Input: part model. Units: mm. Frame: model coordinates. A direction names the side the tool comes from. Coordinates: 2 decimals unless noted, no trailing zeros. Order: outer loops, then holes, each group sorted by start corner. A loop starts at its lowest first (then second) coordinate and runs counter-clockwise, first axis right, second up. Notation, with made-up numbers: (-17.5, 40.25) - (33.5, 40.25) arc R14 cw to (33.5, 55.25) - close; hole circle Ø11 at (61.5, 38.5). An arc over 180 degrees is marked (long way). Answer as CSV lines item,"result". Start each with the question number.
Item 1: Section C-C (z = 1499). Output: boundary loops of the cut face in (x, y), and give its area (3 significant figures).
Item 2: Section A-A (x = 896.5). Output: boundary loops of the cut face in (y, z) (3 decimals), and give its area (3 significant figures).
Item 3: Draft query along Y for faces 1 (the flat face through (1000, 850, 840)), 2 (the flat face through (542, 507, 0)), 3 (the flat face through (546, 900, 49)). Return one class per face: +Y half, -Y half, draft (parallel to the pull), parting line (faces both ways), or undercut.
Item 4: Section B-B (x = 349). Output: boundary loops of the cut face in (y, z) (3 decimals), and give its area (3 significant figures).
Item 5: First-contact query: pin 1 (2 mm diameter, centred on x = 795, z = 531.5, fed in from +Y). Flat tip, straight axial feed; report the tip coordinate or a pass-through.
Item 6: Section D-D (y = 937.5). Output: boundary loops of the cut face in (x, z), and give its area (3 significant figures).
Item 7: Access query for faces 4 (the flat face through (1049, 1200, 1279)), 5 (the flat face through (295, 1008, 51)), 6 (the flat face through (80, 1200, 593)). Directions: +Z, -Z, +X, -X, +Y, -Y. A direction counts if a zero-diameter tool reaches every point of the face in a straight line with its end or side. Return the directions, or none.
Item 8: Material intervals for line 1 along Z through (x, y) = (529, 517); line 2 along Y through (x, z) = (185.5, 950); line 3 along X through (y, z) = (644.5, 1309), sorted ascending.
Autodesk Inventor part; units mm, degrees
ref_plane "YZ Plane" through (0, 0, 0) normal (1, 0, 0) x (0, 1, 0)
ref_plane "XZ Plane" through (0, 0, 0) normal (0, 1, 0) x (-1, 0, 0)
ref_plane "XY Plane" through (0, 0, 0) normal (0, 0, 1) x (1, 0, 0)
sketch "Sketch10" plane through (0, 0, 0) normal (0, 1, 0) x (-1, 0, 0)
  point P0 (0, 0)
sketch "Sketch11" plane through (0, 0, 0) normal (0, 0, 1) x (1, 0, 0)
  point P0 (0, 0)
sketch "Sketch12" plane through (0, 0, 0) normal (0, 0, 1) x (1, 0, 0)
  line L0 (0, 0) -> (1100, 0)
  line L1 (1100, 0) -> (1100, 1200)
  line L2 (1100, 1200) -> (0, 1200)
  line L3 (0, 1200) -> (0, 0)
  dimension "d20" = 1100
  dimension "d21" = 1200
extrude "Extrusion6" add sketch "Sketch12" along normal blind 1700
sketch "Sketch13" plane through (1100, 0, 0) normal (1, 0, 0) x (0, 0, -1)
  line L0 (-100, 100) -> (-1600, 100)
  line L1 (-1600, 100) -> (-1600, 1200)
  line L2 (-1600, 1200) -> (-100, 1200)
  line L3 (-100, 1200) -> (-100, 100)
  point P0 (0, 0)
  dimension "d24" = 1500
extrude "Extrusion7" cut sketch "Sketch13" against normal blind 1000
sketch "Sketch16" plane through (100, 0, 0) normal (1, 0, 0) x (0, 0, -1)
  circle A0 centre (-1499, 200) radius 50
  circle A1 centre (-201, 200) radius 50
  point P0 (0, 0)
  dimension "d34" = 100
  dimension "d35" = 100
extrude "Extrusion10" cut sketch "Sketch16" along normal blind 1200 and the other way blind 200
sketch "Sketch18" plane through (1100, 100, 100) normal (0, 0, 1) x (1, 0, 0)
  line L0 (0, 0) -> (-1000, 0)
  line L1 (-1000, 1100) -> (0, 1100)
  line L2 (0, 0) -> (-100, 0)
  line L3 (-100, 0) -> (-100, 1100)
  line L4 (-100, 1100) -> (0, 1100)
  line L5 (0, 1100) -> (0, 0)
  point P0 (-1100, -100)
  dimension "d43" = 100
extrude "Extrusion12" add sketch "Sketch18" along normal blind 1500
sketch "Sketch19" plane through (0, 0, 1700) normal (0, 0, 1) x (1, 0, 0)
  line L0 (100, 500) -> (1000, 500)
  line L1 (1000, 500) -> (1000, 510)
  line L2 (1000, 510) -> (100, 510)
  line L3 (100, 510) -> (100, 500)
  point P0 (0, 0)
  dimension "d46" = 900
  dimension "d47" = 10
extrude "Extrusion13" add sketch "Sketch19" against normal blind 1700
sketch "Sketch20" plane through (0, 0, 0) normal (0, 0, -1) x (-1, 0, 0)
  line L0 (-805, 1200) -> (-295, 1200)
  line L1 (-295, 1200) -> (-295, 900)
  line L2 (-295, 900) -> (-805, 900)
  line L3 (-805, 900) -> (-805, 1200)
  point P0 (0, 0)
  dimension "d58" = 510
  dimension "d59" = 300
extrude "Extrusion14" cut sketch "Sketch20" against normal blind 1700
sketch "Sketch21" plane through (1100, 1200, 1700) normal (0, 1, 0) x (1, 0, 0)
  line L0 (0, 1700) -> (0, 0)
  line L1 (-1100, 1700) -> (-1100, 0)
  line L2 (0, 470.5254) -> (-1100, 470.5254)
  line L3 (-1100, 470.5254) -> (-1100, 370.5254)
  line L4 (-1100, 370.5254) -> (0, 370.5254)
  line L5 (0, 370.5254) -> (0, 470.5254)
  dimension "d60" = 100
extrude "Extrusion15" add sketch "Sketch21" along normal blind 40
sketch "Sketch22" plane through (1100, 1240, 1700) normal (0, 1, 0) x (1, 0, 0)
  line L0 (-1100, 470.5254) -> (-1100, 370.5254)
  line L1 (0, 370.5254) -> (0, 470.5254)
  line L2 (-1100, 450.525) -> (0, 450.525)
  line L3 (0, 450.525) -> (0, 390.525)
  line L4 (0, 390.525) -> (-1100, 390.525)
  line L5 (-1100, 390.525) -> (-1100, 450.525)
  point P0 (-1100, 1700)
  dimension "d63" = 60
extrude "Extrusion16" cut sketch "Sketch22" against normal blind 40
sketch "Sketch23" plane through (1100, 1240, 1700) normal (0, 1, 0) x (1, 0, 0)
  point P0 (-1100, 1700)
sketch "Sketch25" plane through (1100, 0, 0) normal (1, 0, 0) x (0, 0, -1)
  point P0 (0, 0)
sketch "Sketch27" plane through (0, 0, 0) normal (0, 0, -1) x (-1, 0, 0)
  line L0 (-865, 700) -> (-785, 700)
  line L1 (-785, 700) -> (-785, 600)
  line L2 (-785, 600) -> (-865, 600)
  line L3 (-865, 600) -> (-865, 700)
  line L4 (0, 0) -> (-1100, 0)
  line L5 (-1100, 0) -> (-1100, 1200)
  line L6 (-805, 900) -> (-805, 1200)
  line L7 (-315, 700) -> (-235, 700)
  line L8 (-235, 700) -> (-235, 600)
  line L9 (-235, 600) -> (-315, 600)
  line L10 (-315, 600) -> (-315, 700)
  line L11 (-295, 1200) -> (-295, 900)
  dimension "d77" = 100
  dimension "d78" = 80
  dimension "d79" = 600
  dimension "d81" = 20
  dimension "d82" = 100
  dimension "d83" = 80
  dimension "d84" = 600
  dimension "d85" = 20
extrude "Extrusion17" cut sketch "Sketch27" against normal blind 10
sketch "Sketch28" plane through (0, 1200, 1229.4746) normal (0, 1, 0) x (1, 0, 0)
  line L0 (100, 0) -> (100, 1129.4746)
  line L1 (295, 1129.4746) -> (100, 1129.4746)
  line L2 (100, 1129.4746) -> (100, 878.7986)
  line L3 (100, 878.7986) -> (295, 878.7986)
  line L4 (295, 878.7986) -> (295, 1129.4746)
  point P0 (0, 1229.4746)
  point P1 (100, 1029.4746)
  dimension "d90" = 250.676
extrude "Extrusion18" add sketch "Sketch28" against normal blind 10
sketch "Sketch29" plane through (805, 1200, 0) normal (0, 1, 0) x (1, 0, 0)
  line L0 (0, 0) -> (0, -100)
  line L1 (195, -100) -> (195, -1229.4746)
  line L2 (0, -100) -> (195, -100)
  line L3 (195, -100) -> (195, -350.676)
  line L4 (195, -350.676) -> (0, -350.676)
  line L5 (0, -350.676) -> (0, -100)
  point P0 (-805, 0)
  dimension "d93" = 250.676
extrude "Extrusion19" add sketch "Sketch29" against normal blind 10
sketch "Sketch30" plane through (0, 1200, 0) normal (0, 1, 0) x (1, 0, 0)
  point P0 (0, 0)
fillet "Fillet3" radius 200 2 edges at (952.5, 1200, 0) (147.5, 1200, 0)
sketch "Sketch31" plane through (0, 0, 1700) normal (-1, 0, 0) x (0, 0, 1)
  circle A0 centre (-1499, 200) radius 50
  circle A1 centre (-1499, 200) radius 50
  point P0 (-1700, 0)
extrude "Extrusion20" cut sketch "Sketch31" against normal blind 10000
sketch "Sketch32" plane through (0, 0, 1700) normal (-1, 0, 0) x (0, 0, 1)
  circle A0 centre (-201, 200) radius 50
  circle A1 centre (-201, 200) radius 50
  point P0 (-1700, 0)
extrude "Extrusion21" cut sketch "Sketch32" against normal blind 10000
properties part number "Design" material "Copper"
Determined:
1,outline,"(0, 0) - (1100, 0) - (1100, 150) - (1000, 150) - (1000, 100) - (100, 100) - (100, 150) - (0, 150) - close; (0, 250) - (100, 250) - (100, 500) - (1000, 500) - (1000, 250) - (1100, 250) - (1100, 1200) - (1000, 1200) - (1000, 510) - (100, 510) - (100, 1200) - (0, 1200) - close"
1,area,"319,000 mm^2"
2,outline,"(0, 0) - (1000, 0) arc R200 ccw to (1173.205, 100) - (510, 100) - (510, 1600) - (1200, 1600) - (1200, 1700) - (0, 1700) - close; (1190, 137.55) arc R200 ccw to (1200, 200) - (1200, 350.676) - (1190, 350.676) - close; (1200, 1229.475) - (1240, 1229.475) - (1240, 1249.475) - (1200, 1249.475) - close; (1200, 1309.475) - (1240, 1309.475) - (1240, 1329.475) - (1200, 1329.475) - close; hole (100, 100) - (500, 100) - (500, 1600) - (100, 1600) - close"
2,area,"401,000 mm^2"
3,face 1,"undercut"
3,face 2,"draft"
3,face 3,"+Y half"
4,outline,"(0, 0) - (900, 0) - (900, 100) - (510, 100) - (510, 1600) - (900, 1600) - (900, 1700) - (0, 1700) - close; (1200, 1229.475) - (1240, 1229.475) - (1240, 1249.475) - (1200, 1249.475) - close; (1200, 1309.475) - (1240, 1309.475) - (1240, 1329.475) - (1200, 1329.475) - close; hole (100, 100) - (500, 100) - (500, 1600) - (100, 1600) - close"
4,area,"347,000 mm^2"
5,pin 1,"stops at y = 510"
6,outline,"(0, 0) - (295, 0) - (295, 100) - (100, 100) - (100, 1600) - (295, 1600) - (295, 1700) - (0, 1700) - close; (805, 0) - (1100, 0) - (1100, 1700) - (805, 1700) - (805, 1600) - (1000, 1600) - (1000, 100) - (805, 100) - close"
6,area,"418,000 mm^2"
7,face 4,"+X, -X, +Y"
7,face 5,"+Z, -Z, +Y"
7,face 6,"-Z, +X, -X, +Y"
8,line 1,"z = 0 to 100, 1600 to 1700"
8,line 2,"y = 0 to 100, 500 to 510"
8,line 3,"x = 0 to 100, 1000 to 1100"
